```python
from build123d import *

# Parameters (mm, degrees)
SKETCH1_R           = 34.925
SKETCH1_R_2         = 1.778
BOSS_EXTRUDE1_DEPTH = 6.35
SKETCH2_R           = 3.683
SKETCH2_R_2         = 1.778
BOSS_EXTRUDE2_DEPTH = 6.096
SKETCH3_R           = 3.302
CUT_EXTRUDE1_DEPTH  = 51.935392077
FILLET1_R           = 4.572
SKETCH4_R           = 1.778
CUT_EXTRUDE2_DEPTH  = 51.935392238
SKETCH5_R           = 2.54
CUT_EXTRUDE3_DEPTH  = 51.935392238
FILLET2_R           = 4.7625


with BuildPart() as part:
    # Sketch1 → Boss-Extrude1 (new body)
    with BuildSketch(Plane.XY):
        Circle(SKETCH1_R)
        with Locations((-6.914797213, 6.914797213)):
            Circle(SKETCH1_R_2, mode=Mode.SUBTRACT)
        with Locations((6.914797213, 6.914797213)):
            Circle(SKETCH1_R_2, mode=Mode.SUBTRACT)
        with Locations((6.914797213, -6.914797213)):
            Circle(SKETCH1_R_2, mode=Mode.SUBTRACT)
        with Locations((-6.914797213, -6.914797213)):
            Circle(SKETCH1_R_2, mode=Mode.SUBTRACT)
    extrude(amount=BOSS_EXTRUDE1_DEPTH)

    # Sketch2 → Boss-Extrude2 (add)
    # profile 1 of 2: a face of its own
    with BuildSketch(Plane.XY.offset(6.35)):
        with Locations(Location((0, -28.971875, 0), (0, 0, 180))):
            Circle(SKETCH2_R)
    # profile 2 of 2: a face of its own
    with BuildSketch(Plane.XY.offset(6.35)):
        with BuildLine():
            ThreePointArc((11.864980378, -22.458455882), (0, 25.4), (-11.864980378, -22.458455882))
            ThreePointArc((-11.864980378, -22.458455882), (0, -14.2875), (11.864980378, -22.458455882))
        make_face()
        with Locations((-6.914797213, 6.914797213)):
            Circle(SKETCH2_R_2, mode=Mode.SUBTRACT)
        with Locations((6.914797213, 6.914797213)):
            Circle(SKETCH2_R_2, mode=Mode.SUBTRACT)
    extrude(amount=BOSS_EXTRUDE2_DEPTH)

    # Sketch3 → Cut-Extrude1 (cut, through all)
    with BuildSketch(Plane.XY.offset(12.446)):
        Circle(SKETCH3_R)
    extrude(amount=-CUT_EXTRUDE1_DEPTH, mode=Mode.SUBTRACT)

    # Fillet1
    fillet1_edges = [part.edges().sort_by_distance(p)[0] for p in [
        (-11.864980378, -22.458455882, 9.398),
        (11.864980378, -22.458455882, 9.398),
    ]]
    fillet(fillet1_edges, radius=FILLET1_R)

    # Sketch4 → Cut-Extrude2 (cut, through all)
    with BuildSketch(Plane(origin=(0, 0, 0), x_dir=(-1, 0, 0), z_dir=(0, 0, -1))):
        with Locations((-6.914797213, -6.914797213)):
            Circle(SKETCH4_R)
        with Locations((6.914797213, -6.914797213)):
            Circle(SKETCH4_R)
    extrude(amount=-CUT_EXTRUDE2_DEPTH, mode=Mode.SUBTRACT)

    # Sketch5 → Cut-Extrude3 (cut, through all)
    with BuildSketch(Plane(origin=(0, 0, 0), x_dir=(-1, 0, 0), z_dir=(0, 0, -1))):
        with Locations((-32.004, -6.223)):
            Circle(SKETCH5_R)
    extrude(amount=-CUT_EXTRUDE3_DEPTH, mode=Mode.SUBTRACT)

    # Fillet2
    fillet2_edges = [part.edges().sort_by_distance(p)[0] for p in [
        (34.470468913, -5.616261917, 3.175),
        (34.06339832, -7.709767823, 3.175),
    ]]
    fillet(fillet2_edges, radius=FILLET2_R)


solid = part.part
```
The model under review builds one solid part; all positions refer to its coordinate system, in mm. A direction names the side the tool comes from. Give positions to 0.01 mm unless a question says otherwise; leave off trailing zeros. Write each loop counter-clockwise with the first axis right and the second up, starting at its lowest first coordinate (ties: lowest second). Pieces come first, ordered by that corner, then holes. Notation, with made-up numbers: M 20.5,46.25 L 57.5,46.25 A25 cw 57.5,77.25 Z; hole C 56.25,48 d10. An arc over 180 degrees is marked long. Write item = value, one per line. Start each with the question number.
Q1. Clearance check with flat-ended pins moving along their axes: pin 1 (4 mm diameter, centred on x = 21.5, y = 27, fed in from +Z); pin 2 (4 mm diameter, centred on x = -19, z = 4, fed in from -Y); pin 3 (6 mm diameter, centred on y = 14.5, z = 8.5, fed in from +X). State where each tip first meets the part, or that it passes through.
Q2. We need section B-B (z = 8). Give the number of separate pieces and of enclosed holes in the cut face, plus the area to 3 significant figures.
Q3. For line 1 (Z direction, x = -28.5, y = -10.5); line 2 (X direction, y = -8, z = 4.25); line 3 (X direction, y = 9, z = 1), list the stretches that pass through material, from the lowest coordinate up.
Q4. Machinability: for faces 1 (the face through (3.05, -1.26, 6.31)), 2 (the face through (-0.16, -14.29, 9.36)), which of the approach directions +Z, -Z, +X, -X, +Y, -Y give a long, thin tool a straight path to every point of the face, cutting with its end or side? Answer none if there is none.
Q5. We need section C-C (x = -19.5). State the section outline as (y, z) points, plus the area to 3 significant figures.
Q6. Mouldability with a two-part tool opening along X and no side actions: class faces 3 (the face through (29.5, -5.8, 3.1)), 4 (the face through (0, -7, 0)), 5 (the face through (0.798, -25.376, 9.355)), 6 (the face through (-5.22, 7.45, 6.14)) as released by +X, released by -X, zero draft, split by the parting line, or undercut.
Q7. We need section D-D (y = -28). State the section outline as (x, z) points, plus the area to 3 significant figures.
Result set:
q1.pin_1 = 6.35
q1.pin_2 = -30.51
q1.pin_3 = 32.65
q2.separate_pieces = 2
q2.enclosed_holes = 5
q2.area = 1,800 mm2
q3.line_1 = 0 to 6.35
q3.line_2 = -34 to -8.32, -5.51 to 5.51, 8.32 to 30.19
q3.line_3 = -33.75 to 33.75
q4.face_1 = +Z, -Z
q4.face_2 = +Z
q5.outline = M -28.97,0 L 28.97,0 L 28.97,6.35 L 16.28,6.35 L 16.28,12.45 L -16.28,12.45 L -16.28,6.35 L -28.97,6.35 Z
q5.area = 566 mm2
q6.face_3 = released by +X
q6.face_4 = zero draft
q6.face_5 = split by the parting line
q6.face_6 = undercut
q7.outline = M -20.87,0 L 20.87,0 L 20.87,6.35 L 3.55,6.35 L 3.55,12.45 L -3.55,12.45 L -3.55,6.35 L -20.87,6.35 Z
q7.area = 308 mm2
